```python
from build123d import *

# Parameters (mm, degrees)
SKETCH2_R           = 3.425
BOSS_EXTRUDE2_DEPTH = 3
SKETCH3_W           = 118.4
SKETCH3_H           = 12.75
CUT_EXTRUDE1_DEPTH  = 338.231374578
SKETCH5_R           = 2.625
SKETCH5_R_2         = 4.075
SKETCH5_R_3         = 1.25
SKETCH5_R_4         = 1.625
SKETCH5_R_5         = 7
SKETCH5_W           = 6
SKETCH5_H           = 154
CUT_EXTRUDE2_DEPTH  = 338.231374578


with BuildPart() as part:
    # Sketch2 → Boss-Extrude2 (new body)
    with BuildSketch(Plane.XY):
        with BuildLine():
            Line((25.03035901, 0), (111.286489227, 49.8))
            ThreePointArc((111.286489227, 49.8), (152.858332199, 69.766604349), (181.6, 33.7))
            Line((181.6, 33.7), (181.6, 0))
            Line((181.6, 0), (300, 0))
            Line((300, 0), (300, 145))
            Line((300, 145), (38, 145))
            Line((38, 145), (38, 154))
            Line((38, 154), (19, 154))
            Line((19, 154), (0, 154))
            Line((0, 154), (0, 0))
            Line((0, 0), (25.03035901, 0))
        make_face()
        with Locations((19, 135)):
            Circle(SKETCH2_R, mode=Mode.SUBTRACT)
    extrude(amount=BOSS_EXTRUDE2_DEPTH)

    # Sketch3 → Cut-Extrude1 (cut, through all)
    with BuildSketch(Plane.XY.offset(3)):
        with Locations((240.8, 6.375)):
            Rectangle(SKETCH3_W, SKETCH3_H)
    extrude(amount=-CUT_EXTRUDE1_DEPTH, mode=Mode.SUBTRACT)

    # Sketch5 → Cut-Extrude2 (cut, through all)
    with BuildSketch(Plane.XY.offset(3)):
        with Locations((254.98, 25.75)):
            Circle(SKETCH5_R)
        with Locations((234.98, 25.75)):
            Circle(SKETCH5_R)
        with Locations((288, 130)):
            Circle(SKETCH5_R_2)
        with Locations((288, 138.75)):
            Circle(SKETCH5_R_3)
        with Locations((288, 110.95)):
            Circle(SKETCH5_R_3)
        with Locations((181.6, 72.03)):
            Circle(SKETCH5_R_4)
        with Locations((285.78, 62.92)):
            Circle(SKETCH5_R_4)
        with Locations((52.23, 24.91)):
            Circle(SKETCH5_R_4)
        with Locations((112.84, 59.93)):
            Circle(SKETCH5_R_4)
        with Locations((266.89, 135.99)):
            Circle(SKETCH5_R_4)
        with Locations((128.89, 135.99)):
            Circle(SKETCH5_R_4)
        with Locations((214.98, 34.75)):
            Circle(SKETCH5_R_5)
        with Locations((3, 77)):
            Rectangle(SKETCH5_W, SKETCH5_H)
    extrude(amount=-CUT_EXTRUDE2_DEPTH, mode=Mode.SUBTRACT)


solid = part.part
```
Check sheet for the modelled part. Datum: model origin and axes. Units: mm. Give positions to 0.01 mm unless a question says otherwise; leave off trailing zeros. Loops run counter-clockwise (first coordinate to the right, second up) from the corner with the lowest first, then second, coordinate; pieces in that order, holes last. Notation, with made-up numbers: (13, 29) - (35, 29) arc R10 cw to (35, 41) - close; hole circle Ø7 at (53, -21.5). An arc over 180 degrees is marked (long way). One line per question, with ' | ' between items. Start each with the question number.
1. Cross-section at B-B, the plane z = 2.2. Give the number of separate pieces and of enclosed holes in the cut face, plus the area to 3 significant figures.
2. Cross-section at C-C, the plane y = 47. Enter the section's corners in (x, z).
3. Material ranges on line 1 along X through (y, z) = (139, 0.8); line 2 along X through (y, z) = (59.5, 2.75); line 3 along X through (y, z) = (132, 2.5), recorded low to high. Write a range as [from, to].
4. Cross-section at A-A, the plane x = 19. Enter the section's corners in (y, z) (3 decimals), plus the area to 3 significant figures.
5. Cross-section at D-D, the plane x = 205. Enter the section's corners in (y, z).
6. Gauge pin test, flat ends, axial feed: pin 1 Ø1 at (x, y) = (262, 96) entering from -Z; pin 2 Ø1.5 at (x, z) = (264, 1.5) entering from -Y; pin 3 Ø5 at (x, y) = (288, 130) entering from -Z; pin 4 Ø1 at (x, z) = (181.5, 1.5) entering from +Y. Record the tip position at first contact, or that the pin passes through.
7. Draft check along X on faces 1 (the flat face through (67.55, 24.55, 1.48)), 2 (the flat face through (151, 78, 0)). Enter one of: released by +X, released by -X, zero draft, split by the parting line, or undercut.
Check result:
1) separate pieces: 1 | enclosed holes: 13 | area: 34,400 mm2
2) outline: (6, 0) - (106.44, 0) - (106.44, 3) - (6, 3) - close; (179.13, 0) - (300, 0) - (300, 3) - (179.13, 3) - close
3) line 1: x = [6, 286.78], [289.22, 300] | line 2: x = [6, 111.27], [114.41, 118.08], [171.12, 300] | line 3: x = [6, 17.35], [20.65, 284.45], [291.55, 300]
4) outline: (0, 0) - (131.575, 0) - (131.575, 3) - (0, 3) - close; (138.425, 0) - (154, 0) - (154, 3) - (138.425, 3) - close | area: 441 mm2
5) outline: (12.75, 0) - (145, 0) - (145, 3) - (12.75, 3) - close
6) pin 1: stops at z = 0 | pin 2: stops at y = 12.75 | pin 3: passes through | pin 4: stops at y = 145
7) face 1: undercut | face 2: zero draft
